```python
from build123d import *

# Parameters (mm, degrees)
SKETCH4_W           = 22.098
SKETCH4_H           = 22.098
BOSS_EXTRUDE2_DEPTH = 12.7
FILLET1_R           = 2.54
SKETCH6_R           = 3.175
CUT_EXTRUDE1_DEPTH  = 28.779344935


with BuildPart() as part:
    # Sketch4 → Boss-Extrude2 (new, symmetric)
    with BuildSketch(Plane(origin=(0, 0, 0), x_dir=(1, 0, 0), z_dir=(0, 1, 0))):
        Rectangle(SKETCH4_W, SKETCH4_H)
    extrude(amount=BOSS_EXTRUDE2_DEPTH, both=True)

    # Fillet1
    fillet1_edges = [part.edges().sort_by_distance(p)[0] for p in [
        (11.049, 0, 11.049),
        (-11.049, 0, 11.049),
        (-11.049, 0, -11.049),
        (11.049, 0, -11.049),
    ]]
    fillet(fillet1_edges, radius=FILLET1_R)

    # Sketch6 → Cut-Extrude1 (cut, through all)
    with BuildSketch(Plane(origin=(11.049, 0, 0), x_dir=(0, 0, -1), z_dir=(1, 0, 0))):
        Circle(SKETCH6_R)
    extrude(amount=-CUT_EXTRUDE1_DEPTH, mode=Mode.SUBTRACT)


solid = part.part
```
Read the model definition and answer for the solid it produces. Units are mm, in the model's axes. Coordinates: 2 decimals unless noted, no trailing zeros. Loops run counter-clockwise (first coordinate to the right, second up) from the corner with the lowest first, then second, coordinate; pieces in that order, holes last.
(1) The part is cut by section B-B (y = 0). Determine the outline of the cut face in (x, z) (3 decimals), and give its area (3 significant figures).
Solution:
outline: (-11.049, -8.509) arc R2.54 ccw to (-8.509, -11.049) - (8.509, -11.049) arc R2.54 ccw to (11.049, -8.509) - (11.049, -3.175) - (-11.049, -3.175) - close; (-11.049, 3.175) - (11.049, 3.175) - (11.049, 8.509) arc R2.54 ccw to (8.509, 11.049) - (-8.509, 11.049) arc R2.54 ccw to (-11.049, 8.509) - close
area: 342 mm2
(2) The part is cut by section A-A (z = 0). Determine the outline of the cut face in (x, y) (3 decimals).
Solution:
outline: (-11.049, -12.7) - (11.049, -12.7) - (11.049, -3.175) - (-11.049, -3.175) - close; (-11.049, 3.175) - (11.049, 3.175) - (11.049, 12.7) - (-11.049, 12.7) - close
(3) The mould has two halves that part along Y. Classify faces 1 (the face through (0, 12.7, 0)), 2 (the face through (0, 0, -11.049)), 3 (the face through (0.15, -3.1, 0.69)), 4 (the face through (0, -12.7, 0)): released by +Y, released by -Y, zero draft, split by the parting line, or undercut.
Solution:
face 1: released by +Y
face 2: zero draft
face 3: undercut
face 4: released by -Y
(4) The part is cut by section C-C (x = -2). Determine the outline of the cut face in (y, z) (3 decimals), and give its area (3 significant figures).
Solution:
outline: (-12.7, -11.049) - (12.7, -11.049) - (12.7, 11.049) - (-12.7, 11.049) - close; hole circle Ø6.35 at (0, 0)
area: 530 mm2
(5) Consider line 1 along Y through (x, z) = (4.75, 0) (3 decimals); line 2 along Y through (x, z) = (0.25, -0.75); line 3 along Z through (x, y) = (7.75, 2.25). Determine where each line is inside the solid, lowest interval first.
Solution:
line 1: y = -12.7 to -3.175, 3.175 to 12.7
line 2: y = -12.7 to -3.09, 3.09 to 12.7
line 3: z = -11.05 to -2.24, 2.24 to 11.05
(6) A flat-ended cylindrical pin translates along its axis: pin 1 Ø4 at (y, z) = (0, 0) entering from +X. Find the tip coordinate at first contact, or state that the pin passes through.
Solution:
pin 1: passes through
